Verification items for the finished model (mm, model axes). A direction names the side the tool comes from. Round coordinates to 2 decimals unless told otherwise and drop trailing zeros. Write each loop counter-clockwise with the first axis right and the second up, starting at its lowest first coordinate (ties: lowest second). Pieces come first, ordered by that corner, then holes.
from build123d import *

# Parameters (mm, degrees)
SKETCH1_W           = 76
SKETCH1_H           = 40
SKETCH1_R           = 2.75
BOSS_EXTRUDE1_DEPTH = 4
SKETCH2_W           = 50
SKETCH2_H           = 50
SKETCH2_W_2         = 30
SKETCH2_H_2         = 17
BOSS_EXTRUDE2_DEPTH = 4
SKETCH3_R           = 2.75
CUT_EXTRUDE1_DEPTH  = 4
FILLET1_R           = 4


with BuildPart() as part:
    # Sketch1 → Boss-Extrude1 (new body)
    with BuildSketch(Plane(origin=(0, 0, 0), x_dir=(1, 0, 0), z_dir=(0, 1, 0))):
        with Locations((0, -5)):
            Rectangle(SKETCH1_W, SKETCH1_H)
        with Locations((-30, 7)):
            Circle(SKETCH1_R, mode=Mode.SUBTRACT)
        with Locations((30, 7)):
            Circle(SKETCH1_R, mode=Mode.SUBTRACT)
        with Locations((-30, -17)):
            Circle(SKETCH1_R, mode=Mode.SUBTRACT)
        with Locations((30, -17)):
            Circle(SKETCH1_R, mode=Mode.SUBTRACT)
    extrude(amount=BOSS_EXTRUDE1_DEPTH)

    # Sketch2 → Boss-Extrude2 (add)
    with BuildSketch(Plane(origin=(0, 4, 0), x_dir=(1, 0, 0), z_dir=(0, 1, 0))):
        with Locations((0, -50)):
            Rectangle(SKETCH2_W, SKETCH2_H)
        with Locations((0, 23.5)):
            Rectangle(SKETCH2_W_2, SKETCH2_H_2)
    extrude(amount=-BOSS_EXTRUDE2_DEPTH)

    # Sketch3 → Cut-Extrude1 (cut)
    with BuildSketch(Plane(origin=(0, 4, 0), x_dir=(1, 0, 0), z_dir=(0, 1, 0))):
        with Locations((0, 23.5)):
            Circle(SKETCH3_R)
        with Locations((0, -7)):
            Circle(SKETCH3_R)
        with Locations((-10, -40)):
            Circle(SKETCH3_R)
        with Locations((10, -40)):
            Circle(SKETCH3_R)
        with Locations((-10, -60)):
            Circle(SKETCH3_R)
        with Locations((10, -60)):
            Circle(SKETCH3_R)
    extrude(amount=-CUT_EXTRUDE1_DEPTH, mode=Mode.SUBTRACT)

    # Fillet1
    fillet1_edges = [part.edges().sort_by_distance(p)[0] for p in [
        (-25, 2, 75),
        (25, 2, 75),
        (25, 2, 25),
        (38, 2, 25),
        (38, 2, -15),
        (-38, 2, -15),
        (-38, 2, 25),
        (-25, 2, 25),
        (15, 2, -15),
        (15, 2, -32),
        (-15, 2, -32),
        (-15, 2, -15),
    ]]
    fillet(fillet1_edges, radius=FILLET1_R)


solid = part.part
Q1. Depth check by flat-ended pin: P1, Ø1.2, axis at x = -29.5, y = 1.5, coming from the -Z side; P2, Ø9, axis at x = 0, z = 7, coming from the -Y side; P3, Ø2, axis at x = 30.5, y = 3, coming from the +Z side; P4, Ø2, axis at y = 1.5, z = -25.5, coming from the -X side. Enter the tip coordinate at first touch or a pass-through.
Recorded:
P1: stops at z = -15
P2: stops at y = 0
P3: stops at z = 25
P4: stops at x = -15
Q2. Sectioned sample at C-C (y = 1.3). Give the number of separate pieces and of enclosed holes in the cut face, plus the area to 3 significant figures.
Recorded:
separate pieces: 1
enclosed holes: 10
area: 5,800 mm2
Q3. Sectioned sample at D-D (z = 65.5). Enter the section's corners in (x, y), plus the area to 3 significant figures.
Recorded:
outline: (-25, 0) - (25, 0) - (25, 4) - (-25, 4) - close
area: 200 mm2
Q4. Tool access check on faces 1 (the flat face through (-25, 2, 50)), 2 (the flat face through (-15, 2, -23)), 3 (the flat face through (26, 2, -15)). Record the directions out of +Z, -Z, +X, -X, +Y, -Y that give a thin tool (end or side, any length) a straight path to the whole face; none if there is none.
Recorded:
face 1: +Z, -X, +Y, -Y
face 2: -Z, -X, +Y, -Y
face 3: -Z, +X, +Y, -Y
Q5. Sectioned sample at B-B (x = 1). Enter the section's corners in (y, z), plus the area to 3 significant figures.
Recorded:
outline: (0, -32) - (4, -32) - (4, -26.06) - (0, -26.06) - close; (0, -20.94) - (4, -20.94) - (4, 4.44) - (0, 4.44) - close; (0, 9.56) - (4, 9.56) - (4, 75) - (0, 75) - close
area: 387 mm2
Q6. Material ranges on line 1 along Z through (x, y) = (-30, 2.3); line 2 along Z through (x, y) = (0, 1.9); line 3 along X through (y, z) = (2.2, 60), recorded low to high.
Recorded:
line 1: z = -15 to -9.75, -4.25 to 14.25, 19.75 to 25
line 2: z = -32 to -26.25, -20.75 to 4.25, 9.75 to 75
line 3: x = -25 to -12.75, -7.25 to 7.25, 12.75 to 25
Q7. Sectioned sample at A-A (z = 17). Enter the section's corners in (x, y), plus the area to 3 significant figures.
Recorded:
outline: (-38, 0) - (-32.75, 0) - (-32.75, 4) - (-38, 4) - close; (-27.25, 0) - (27.25, 0) - (27.25, 4) - (-27.25, 4) - close; (32.75, 0) - (38, 0) - (38, 4) - (32.75, 4) - close
area: 260 mm2
